Source: three-view drawing plus pictorial views. Frame: mm from the lowest corner of the part. A direction names the side the tool comes from. Give positions to 0.01 mm unless a question says otherwise; leave off trailing zeros. Loops run counter-clockwise (first coordinate to the right, second up) from the corner with the lowest first, then second, coordinate; pieces in that order, holes last. Notation, with made-up numbers: (54, 61) - (75, 61) arc R30 ccw to (75, 99) - close; hole circle Ø4 at (78.5, 56.5). An arc over 180 degrees is marked (long way). Answer as a JSON object with one key per item and string values.
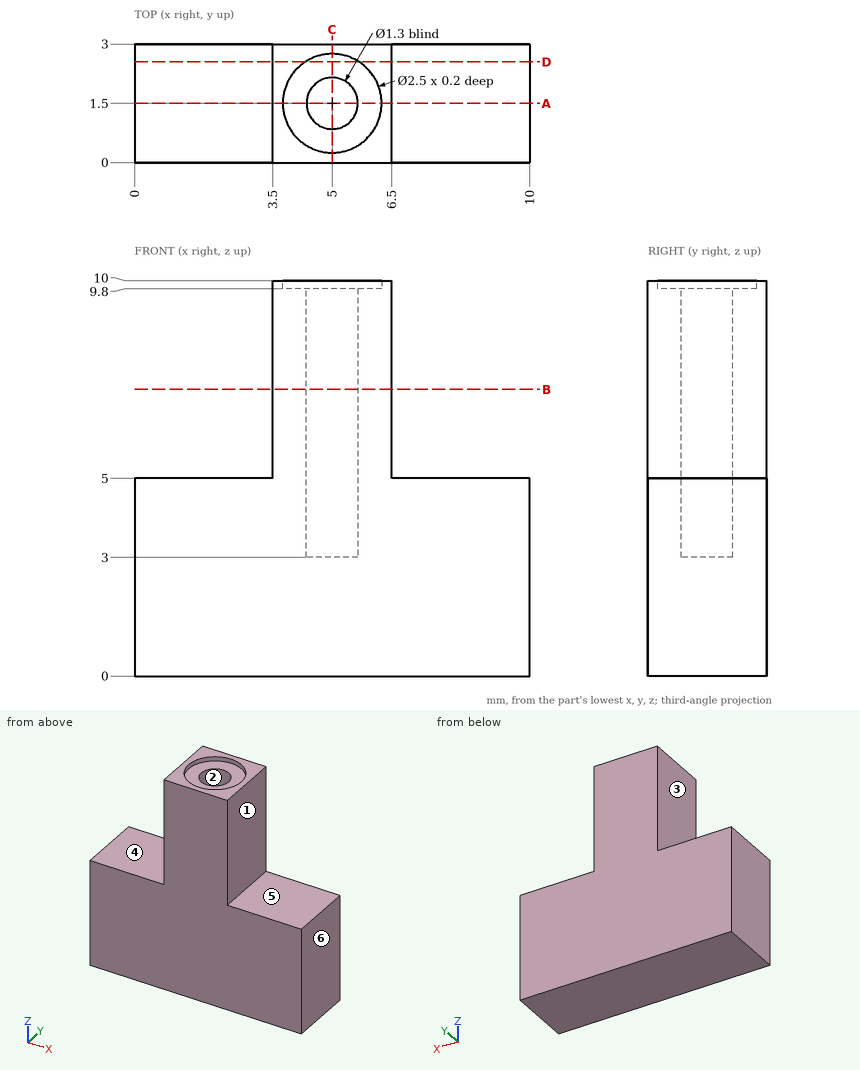
Item 1: Cut plane D-D (y = 2.55). Return loops of the section in (x, z).
Geometry check:
{"outline": "(0, 0) - (10, 0) - (10, 5) - (6.5, 5) - (6.5, 10) - (5.68, 10) - (5.68, 9.8) - (4.32, 9.8) - (4.32, 10) - (3.5, 10) - (3.5, 5) - (0, 5) - close"}
Item 2: Access query for the marked faces 4, 5 and 6. Directions: +Z, -Z, +X, -X, +Y, -Y. A direction counts if a zero-diameter tool reaches every point of the face in a straight line with its end or side. Return the directions, or none.
Geometry check:
{"face 4": "+Z, -X, +Y, -Y", "face 5": "+Z, +X, +Y, -Y", "face 6": "+Z, -Z, +X, +Y, -Y"}
Item 3: Cut plane A-A (y = 1.5). Return loops of the section in (x, z).
Geometry check:
{"outline": "(0, 0) - (10, 0) - (10, 5) - (6.5, 5) - (6.5, 10) - (6.25, 10) - (6.25, 9.8) - (5.65, 9.8) - (5.65, 3) - (4.35, 3) - (4.35, 9.8) - (3.75, 9.8) - (3.75, 10) - (3.5, 10) - (3.5, 5) - (0, 5) - close"}
Item 4: Cut plane C-C (x = 5). Return loops of the section in (y, z).
Geometry check:
{"outline": "(0, 0) - (3, 0) - (3, 10) - (2.75, 10) - (2.75, 9.8) - (2.15, 9.8) - (2.15, 3) - (0.85, 3) - (0.85, 9.8) - (0.25, 9.8) - (0.25, 10) - (0, 10) - close"}
Item 5: Mould query, pull axis X, two halves, no side actions, for the marked faces 1, 2 and 3. Classes: released by +X, released by -X, zero draft, split by the parting line, or undercut.
Geometry check:
{"face 1": "released by +X", "face 2": "undercut", "face 3": "released by -X"}
Item 6: Material intervals for line 1 (Y direction, x = 5, z = 6.5); line 2 (Z direction, x = 8.75, y = 1.9); line 3 (X direction, y = 1.2, z = 9), sorted ascending. Write a range as [from, to].
Geometry check:
{"line 1": "y = [0, 0.85], [2.15, 3]", "line 2": "z = [0, 5]", "line 3": "x = [3.5, 4.42], [5.58, 6.5]"}
Item 7: Contact query for flat-ended pins moving along their axis: P1, Ø0.6, axis at x = 5, y = 1.5, coming from the +Z side; P2, Ø5, axis at x = 3.5, z = 5, coming from the -Y side; P3, Ø1.5, axis at x = 8, y = 1, coming from the +Z side. Output: stop coordinate, or through.
Geometry check:
{"P1": "stops at z = 3", "P2": "stops at y = 0", "P3": "stops at z = 5"}
Item 8: Cut plane B-B (z = 7.25). Return loops of the section in (x, y), then the cut area to 3 significant figures.
Geometry check:
{"outline": "(3.5, 0) - (6.5, 0) - (6.5, 3) - (3.5, 3) - close; hole circle Ø1.3 at (5, 1.5)", "area": "7.67 mm2"}
